```python
from build123d import *

# Parameters (mm, degrees)
F0_W     = 40
F0_H     = 30
F0_R     = 1.75
F0_W_2   = 14
F0_H_2   = 5
F0_W_3   = 5
F0_H_3   = 11
F0_R_2   = 3.5
F1_DEPTH = 6
F2_DEPTH = 2
F4_DEPTH = 3
F5_R     = 5


with BuildPart() as f1:
    # F0 (on Front) → F1 (new body)
    with BuildSketch(Plane.XZ):
        Rectangle(F0_W, F0_H)
        with Locations((-16.5, -11)):
            Circle(F0_R, mode=Mode.SUBTRACT)
        with Locations((-7, -5)):
            Rectangle(F0_W_2, F0_H_2, mode=Mode.SUBTRACT)
        with Locations((2.5, -11)):
            Circle(F0_R, mode=Mode.SUBTRACT)
        with Locations((8.5, -5.5)):
            Rectangle(F0_W_3, F0_H_3, mode=Mode.SUBTRACT)
        with Locations((-10, 8)):
            Circle(F0_R_2, mode=Mode.SUBTRACT)
        with Locations((10, 8)):
            Circle(F0_R_2, mode=Mode.SUBTRACT)
        with Locations((-7, -5)):
            Rectangle(F0_W_2, F0_H_2)
        with Locations((8.5, -5.5)):
            Rectangle(F0_W_3, F0_H_3)
        with Locations((10, 8)):
            Circle(F0_R_2)
        with Locations((10, 8)):
            Circle(F0_R, mode=Mode.SUBTRACT)
        with Locations((-10, 8)):
            Circle(F0_R_2)
        with Locations((-10, 8)):
            Circle(F0_R, mode=Mode.SUBTRACT)
    extrude(amount=-F1_DEPTH)

    # F0 (on Front) → F2 (cut)
    with BuildSketch(Plane.XZ):
        with Locations((8.5, -5.5)):
            Rectangle(F0_W_3, F0_H_3)
        with Locations((-7, -5)):
            Rectangle(F0_W_2, F0_H_2)
        with Locations((-10, 8)):
            Circle(F0_R_2)
        with Locations((-10, 8)):
            Circle(F0_R, mode=Mode.SUBTRACT)
        with Locations((10, 8)):
            Circle(F0_R_2)
        with Locations((10, 8)):
            Circle(F0_R, mode=Mode.SUBTRACT)
    extrude(amount=-F2_DEPTH, mode=Mode.SUBTRACT)

    # F3 (on face) → F4 (cut)
    with BuildSketch(Plane(origin=(0, 6, 0), x_dir=(-1, 0, 0), z_dir=(0, 1, 0))):
        Polygon((-2.5, -7.535898), (-5.5, -9.267949), (-5.5, -12.732051), (-2.5, -14.464102), (0.5, -12.732051), (0.5, -9.267949), align=None)
        Polygon((13.5, -9.267949), (13.5, -12.732051), (16.5, -14.464102), (19.5, -12.732051), (19.5, -9.267949), (16.5, -7.535898), align=None)
    extrude(amount=-F4_DEPTH, mode=Mode.SUBTRACT)

    # F5
    f5_edges = [f1.edges().sort_by_distance(p)[0] for p in [
        (20, 3, 15),
        (-20, 3, 15),
    ]]
    fillet(f5_edges, radius=F5_R)


solid = f1.part
```
Geometry: final body of the model. Coordinates: model frame, mm. A direction names the side the tool comes from. Give positions to 0.01 mm unless a question says otherwise; leave off trailing zeros. Order: outer loops, then holes, each group sorted by start corner. A loop starts at its lowest first (then second) coordinate and runs counter-clockwise, first axis right, second up. Notation, with made-up numbers: M 89,81 L 133,81 A20 ccw 133,97 Z; hole C 17.5,63.5 d6. An arc over 180 degrees is marked long. Answer as CSV lines item,"result". Start each with the question number.
1) Cut plane D-D (y = 5). Output: boundary loops of the cut face in (x, z), then the cut area to 3 significant figures.
2) Set-up query: faces 4 (the cylindrical face through (2.272, 1.479, -9.265)), 5 (the flat face through (8, 1, 0)), 6 (the flat face through (-15, 4.5, -13.6)). Return all of +Z, -Z, +X, -X, +Y, -Y with unobstructed straight access to the full face (end or side cutting, diameter ignored); none if empty.
3) Line query: line 1 (X direction, y = 1.35, z = -5.75); line 2 (Z direction, x = -10, y = 1.1); line 3 (X direction, y = 4.65, z = 7.25). Output: solid intervals per line, ascending. Write a range as from..to.
4) Cut plane B-B (y = 1.05). Output: boundary loops of the cut face in (x, z), then the cut area to 3 significant figures.
5) First-contact query: P1, Ø4.5, axis at x = 10, z = 8, coming from the -Y side. Flat tip, straight axial feed; report the tip coordinate or a pass-through.
6) Mould query, pull axis Z, two halves, no side actions, for faces 1 (the flat face through (0, 3, 15)), 2 (the flat face through (5.5, 5, -11)), 3 (the flat face through (0, 6, 0)). Classes: +Z half, -Z half, draft (parallel to the pull), parting line (faces both ways), or undercut.
7) Cut plane A-A (x = 10). Output: boundary loops of the cut face in (y, z).
8) Cut plane C-C (z = 8). Output: boundary loops of the cut face in (x, y).
Findings below:
1,outline,"M -20,-15 L 20,-15 L 20,10 A5 ccw 15,15 L -15,15 A5 ccw -20,10 Z; hole M -19.5,-12.73 L -16.5,-14.46 L -13.5,-12.73 L -13.5,-9.27 L -16.5,-7.54 L -19.5,-9.27 Z; hole C -10,8 d3.5; hole M -0.5,-12.73 L 2.5,-14.46 L 5.5,-12.73 L 5.5,-9.27 L 2.5,-7.54 L -0.5,-9.27 Z; hole C 10,8 d3.5"
1,area,"1,110 mm²"
2,face 4,"+Y, -Y"
2,face 5,"-Y"
2,face 6,"+Y"
3,line 1,"x = -20..-14, 0..6, 11..20"
3,line 2,"z = -15..-7.5, -2.5..4.5, 11.5..15"
3,line 3,"x = -20..-11.58, -8.42..8.42, 11.58..20"
4,outline,"M -20,-15 L 20,-15 L 20,10 A5 ccw 15,15 L -15,15 A5 ccw -20,10 Z; hole C -16.5,-11 d3.5; hole M -14,-7.5 L 0,-7.5 L 0,-2.5 L -14,-2.5 Z; hole C -10,8 d7; hole C 2.5,-11 d3.5; hole M 6,-11 L 11,-11 L 11,0 L 6,0 Z; hole C 10,8 d7"
4,area,"968 mm²"
5,P1,"stops at y = 2"
6,face 1,"+Z half"
6,face 2,"undercut"
6,face 3,"draft"
7,outline,"M 0,-15 L 6,-15 L 6,6.25 L 2,6.25 L 2,4.5 L 0,4.5 L 0,0 L 2,0 L 2,-11 L 0,-11 Z; M 0,11.5 L 2,11.5 L 2,9.75 L 6,9.75 L 6,15 L 0,15 Z"
8,outline,"M -20,0 L -13.5,0 L -13.5,2 L -11.75,2 L -11.75,6 L -20,6 Z; M -8.25,2 L -6.5,2 L -6.5,0 L 6.5,0 L 6.5,2 L 8.25,2 L 8.25,6 L -8.25,6 Z; M 11.75,2 L 13.5,2 L 13.5,0 L 20,0 L 20,6 L 11.75,6 Z"
